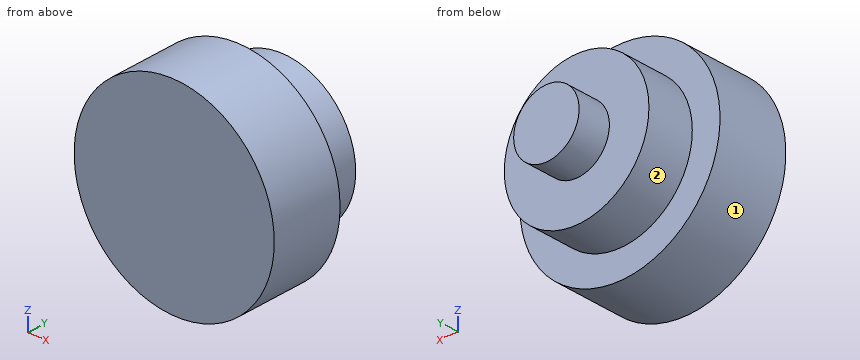
from build123d import *

# Parameters (mm, degrees)
F0_R     = 65.064224
F1_DEPTH = 46.824317
F2_R     = 47.040122
F3_DEPTH = 77.640906
F4_R     = 21.28271
F5_DEPTH = 99.144967


with BuildPart() as f1:
    # F0 (on Front) → F1 (new body)
    with BuildSketch(Plane.XZ):
        Circle(F0_R)
    extrude(amount=-F1_DEPTH)

    # F2 (on Front) → F3 (join)
    with BuildSketch(Plane.XZ):
        Circle(F2_R)
    extrude(amount=-F3_DEPTH)

    # F4 (on Front) → F5 (join)
    with BuildSketch(Plane.XZ):
        Circle(F4_R)
    extrude(amount=-F5_DEPTH)


solid = f1.part
Here's how the part is built. I have some questions about the finished solid (model axes, mm). Face numbers are marked on the shaded views. A direction names the side the tool comes from. Round coordinates to 2 decimals unless told otherwise and drop trailing zeros. Write each loop counter-clockwise with the first axis right and the second up, starting at its lowest first coordinate (ties: lowest second). Pieces come first, ordered by that corner, then holes.
1. Suppose I cut it at D-D (z = 39). List the corners of the cut face in (x, y) for me.
2. Suppose I cut it at C-C (y = 24). List the corners of the cut face in (x, z) for me.
3. Suppose I cut it at A-A (z = 0). List the corners of the cut face in (x, y) for me, and give its area (3 significant figures).
4. Will these pins go through, and if not, where does the flat tip stop? pin 1 Ø1 at (y, z) = (25, -43.5) entering from +X; pin 2 Ø10 at (y, z) = (28, 35.5) entering from +X; pin 3 Ø10 at (x, z) = (27.5, 35.5) entering from +Y.
5. Suppose I cut it at B-B (x = 0). List the corners of the cut face in (y, z) for me, and give its area (3 significant figures).
6. I need wall thicknesses on L1, parallel to Y at x = -46, z = 22; L2, parallel to Y at x = 31.5, z = 13.5; L3, parallel to Z at x = 6.5, y = 33.5. Which ranges of each line are inside material? Lowest first, please.
7. For the marked faces 1 and 2, which set-ups out of +Z, -Z, +X, -X, +Y, -Y let a thin tool reach every point of the face, with its end or its side?
Answer sheet:
1. outline: (-52.08, 0) - (52.08, 0) - (52.08, 46.82) - (26.3, 46.82) - (26.3, 77.64) - (-26.3, 77.64) - (-26.3, 46.82) - (-52.08, 46.82) - close
2. outline: circle Ø130.13 at (0, 0)
3. outline: (-65.06, 0) - (65.06, 0) - (65.06, 46.82) - (47.04, 46.82) - (47.04, 77.64) - (21.28, 77.64) - (21.28, 99.14) - (-21.28, 99.14) - (-21.28, 77.64) - (-47.04, 77.64) - (-47.04, 46.82) - (-65.06, 46.82) - close
3. area: 9,910 mm2
4. pin 1: stops at x = 48.83
4. pin 2: stops at x = 57.47
4. pin 3: stops at y = 77.64
5. outline: (0, -65.06) - (46.82, -65.06) - (46.82, -47.04) - (77.64, -47.04) - (77.64, -21.28) - (99.14, -21.28) - (99.14, 21.28) - (77.64, 21.28) - (77.64, 47.04) - (46.82, 47.04) - (46.82, 65.06) - (0, 65.06) - close
5. area: 9,910 mm2
6. L1: y = 0 to 46.82
6. L2: y = 0 to 77.64
6. L3: z = -64.74 to 64.74
7. face 1: +Y, -Y
7. face 2: +Y
